from build123d import *

# Parameters (mm, degrees)
F0_R          = 27
F0_R_2        = 13.50515
F1_DEPTH      = 25
F2_R          = 9.377807
F4_R          = 4.220987
F5_DEPTH      = 30
F5_DEPTH_BACK = 30


with BuildPart() as f1:
    # F0 (on Top) → F1 (new body)
    with BuildSketch(Plane.XY):
        Circle(F0_R)
        Circle(F0_R_2, mode=Mode.SUBTRACT)
    extrude(amount=F1_DEPTH)

    # F2 (on Right) → F3 (revolve)
    with BuildSketch(Plane.YZ):
        with Locations((-27, 25)):
            Circle(F2_R)
    revolve(axis=Axis((0, 0, 0), (0, 0, -1)))

    # F4 (on Front) → F5 (cut, two sides)
    with BuildSketch(Plane.XZ) as f5_sk:
        with Locations((5.346159, 9.811127)):
            Circle(F4_R)
    extrude(amount=F5_DEPTH, mode=Mode.SUBTRACT)
    extrude(f5_sk.sketch, amount=-F5_DEPTH_BACK, mode=Mode.SUBTRACT)


solid = f1.part
Design review of the part built by this model. Coordinates are the model's own, in mm. A direction names the side the tool comes from. Round coordinates to 2 decimals unless told otherwise and drop trailing zeros. Write each loop counter-clockwise with the first axis right and the second up, starting at its lowest first coordinate (ties: lowest second). Pieces come first, ordered by that corner, then holes.
Item 1: Consider section A-A on x = 0. Give the boundary of the cut face in (y, z), and give its area (3 significant figures).
Item 2: Wall thickness on L1, parallel to Y at x = 0, z = 7; L2, parallel to Z at x = 15, y = 2; L3, parallel to X at y = 16, z = 29.5: over which ranges is each line inside the solid? List them lowest first.
Item 3: For pin 1 Ø5 at (x, y) = (12, -6.5) entering from -Z; pin 2 Ø10 at (x, z) = (21.5, 21) entering from -Y; pin 3 Ø8 at (y, z) = (-7.5, 16.5) entering from -X; pin 4 Ø7 at (x, z) = (5.35, 9.81) entering from +Y, all flat-tipped, find the tip position at first contact; note any pin that passes through.
Item 4: For faces 1 (the cylindrical face through (-5.85, -26.36, 7.7)), 2 (the cylindrical face through (9.37, -20.07, 11.08)), list the 3-axis set-ups (+Z, -Z, +X, -X, +Y, -Y) from which the entire face can be reached by the end or side of a thin tool; tool diameter is ignored.
Item 5: Draft analysis for pull direction Z (two halves, no side actions). For faces 3 (the flat face through (9.1, -10.4, 25)), 4 (the cylindrical face through (9.37, 20.07, 11.08)), 5 (the flat face through (-6.4, 12.4, 0)), state which applies: released by +Z, released by -Z, zero draft, split by the parting line, or undercut.
Check values:
1. outline: (-27, 0) - (-13.51, 0) - (-13.51, 25) - (-17.62, 25) arc R9.38 ccw (long way) to (-27, 15.62) - close; (13.51, 0) - (27, 0) - (27, 15.62) arc R9.38 ccw (long way) to (17.62, 25) - (13.51, 25) - close
1. area: 1,090 mm2
2. L1: y = -27 to -13.51, 13.51 to 27
2. L2: z = 0 to 25
2. L3: x = -31.38 to -9.82, 9.82 to 31.38
3. pin 1: stops at z = 0
3. pin 2: stops at y = -31.96
3. pin 3: stops at x = -34.55
3. pin 4: passes through
4. face 1: -Z
4. face 2: +Y, -Y
5. face 3: released by +Z
5. face 4: undercut
5. face 5: released by -Z
